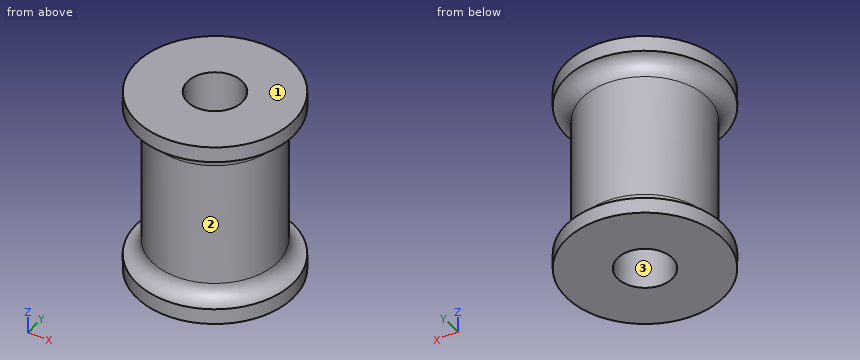
from build123d import *

# Parameters (mm, degrees)
SKETCH1_R           = 10
BOSS_EXTRUDE1_DEPTH = 24
SKETCH3_R           = 3.5
CUT_EXTRUDE1_DEPTH  = 24


with BuildPart() as part:
    # Sketch1 → Boss-Extrude1 (new body)
    with BuildSketch(Plane.XY):
        Circle(SKETCH1_R)
    extrude(amount=BOSS_EXTRUDE1_DEPTH)

    # Sketch2 → Cut-Revolve1 (revolve, cut)
    with BuildSketch(Plane(origin=(0, 0, 0), x_dir=(0, 0, -1), z_dir=(1, 0, 0)), mode=Mode.PRIVATE) as cut_revolve1_sk:
        with BuildLine():
            Line((-22, 10), (-2, 10))
            ThreePointArc((-2, 10), (-2.585786438, 8.585786438), (-4, 8))
            Line((-4, 8), (-20, 8))
            ThreePointArc((-20, 8), (-21.414213562, 8.585786438), (-22, 10))
        make_face()
    revolve(cut_revolve1_sk.sketch.rotate(Axis((0, 0, -0.3), (0, 0, 1)), 90), axis=Axis((0, 0, -0.3), (0, 0, 1)), mode=Mode.SUBTRACT)

    # Sketch3 → Cut-Extrude1 (cut)
    with BuildSketch(Plane(origin=(0, 0, 0), x_dir=(-1, 0, 0), z_dir=(0, 0, -1))):
        Circle(SKETCH3_R)
    extrude(amount=-CUT_EXTRUDE1_DEPTH, mode=Mode.SUBTRACT)


solid = part.part
The listing builds one solid part. Answer for the finished solid, in the listing's coordinates (mm). Face numbers are marked on the shaded views. Coordinates: 2 decimals unless noted, no trailing zeros. Write each loop counter-clockwise with the first axis right and the second up, starting at its lowest first coordinate (ties: lowest second). Pieces come first, ordered by that corner, then holes. Notation, with made-up numbers: M 40,-36.75 L 77,-36.75 A13 cw 77,-13.75 Z; hole C 50.5,64 d8. An arc over 180 degrees is marked long. Write each question's results on one line, items separated by ' | '.
Item 1: The part is cut by section A-A on y = 0. Determine the outline of the cut face in (x, z), and give its area (3 significant figures).
Answer below:
outline: M -10,0 L -3.5,0 L -3.5,24 L -10,24 L -10,22 A2 cw -8,20 L -8,4 A2 cw -10,2 Z; M 3.5,0 L 10,0 L 10,2 A2 cw 8,4 L 8,20 A2 cw 10,22 L 10,24 L 3.5,24 Z | area: 235 mm2
Item 2: For a pull along X with two mould halves and no side action, classify the marked faces 1, 2 and 3 as released by +X, released by -X, zero draft, split by the parting line, or undercut.
Answer below:
face 1: zero draft | face 2: split by the parting line | face 3: undercut
Item 3: The part is cut by section C-C on z = 8.25. Determine the outline of the cut face in (x, y).
Answer below:
outline: C 0,0 d16; hole C 0,0 d7
Item 4: Given P1, Ø3, axis at x = 3.5, z = 8.5, coming from the -Y side; P2, Ø5, axis at y = -2, z = 15, coming from the -X side; P3, Ø10, axis at y = 6.5, z = 5.5, coming from the +X side, each flat-ended and moving along its own axis, determine where each tip first touches the part or whether it passes through.
Answer below:
P1: y = -7.75 | P2: x = -8 | P3: x = 9.56
Item 5: Consider probe 1 along Y at (x, z) = (0, 9); probe 2 along Z at (x, y) = (-8.25, -4); probe 3 along Y at (x, z) = (-1, 19). Determine where each line is inside the solid, lowest interval first. Write a range as [from, to].
Answer below:
probe 1: [-8, -3.5], [3.5, 8] | probe 2: [0, 2.18], [21.82, 24] | probe 3: [-7.94, -3.35], [3.35, 7.94]
